```python
from build123d import *

# Parameters (mm, degrees)
SKETCH1_R           = 2.6
BOSS_EXTRUDE1_DEPTH = 5


with BuildPart() as part:
    # Sketch1 → Boss-Extrude1 (new body)
    with BuildSketch(Plane.XY):
        with BuildLine():
            Line((-144.395039413, -128.65), (-89.395039413, -128.65))
            Line((-89.395039413, -128.65), (-89.395039413, -113.602732617))
            add(Edge.make_bspline(
                [(-89.395039413, -113.602732617), (-96.831752604, -104.34489473), (-107.166514085, -96.997462442), (-119.395039413, -95.65)],
                knots=[0, 0, 0, 0, 1, 1, 1, 1], degree=3))
            Line((-119.395039413, -95.65), (-129.395039413, -95.65))
            Line((-129.395039413, -95.65), (-129.395039413, -90.65))
            Line((-129.395039413, -90.65), (-149.395039413, -90.65))
            Line((-149.395039413, -90.65), (-149.395039413, -95.65))
            Line((-149.395039413, -95.65), (-159.395039413, -95.65))
            Line((-159.395039413, -95.65), (-159.395039413, -90.65))
            Line((-159.395039413, -90.65), (-179.395039413, -90.65))
            Line((-179.395039413, -90.65), (-179.395039413, -95.65))
            add(Edge.make_bspline(
                [(-179.395039413, -95.65), (-181.601038643, -112.074647686), (-182.084492752, -128.65)],
                knots=[0, 0, 0, 1, 1, 1], degree=2))
            add(Edge.make_bspline(
                [(-182.084492752, -128.65), (-182.242729915, -142.32211305), (-189.395039413, -154.585895155)],
                knots=[0, 0, 0, 1, 1, 1], degree=2))
            Line((-189.395039413, -154.585895155), (-189.395039413, -164.35))
            Line((-189.395039413, -164.35), (-179.395039413, -164.35))
            Line((-179.395039413, -164.35), (-179.395039413, -169.35))
            Line((-179.395039413, -169.35), (-159.395039413, -169.35))
            Line((-159.395039413, -169.35), (-159.395039413, -164.35))
            Line((-159.395039413, -164.35), (-149.395039413, -164.35))
            Line((-149.395039413, -164.35), (-149.395039413, -169.35))
            Line((-149.395039413, -169.35), (-129.395039413, -169.35))
            Line((-129.395039413, -169.35), (-129.395039413, -164.35))
            Line((-129.395039413, -164.35), (-119.395039413, -164.35))
            add(Edge.make_bspline(
                [(-89.395039413, -146.397267383), (-96.831752604, -155.65510527), (-107.166514085, -163.002537558), (-119.395039413, -164.35)],
                knots=[0, 0, 0, 0, 1, 1, 1, 1], degree=3))
            Line((-89.395039413, -146.397267383), (-89.395039413, -131.35))
            Line((-89.395039413, -131.35), (-144.395039413, -131.35))
            Line((-144.395039413, -131.35), (-144.395039413, -128.65))
        make_face()
        with Locations((-104.860428981, -112.5)):
            Circle(SKETCH1_R, mode=Mode.SUBTRACT)
        with Locations((-104.860428981, -147.5)):
            Circle(SKETCH1_R, mode=Mode.SUBTRACT)
    extrude(amount=BOSS_EXTRUDE1_DEPTH)


solid = part.part
```
Read the model definition and answer for the solid it produces. Units are mm, in the model's axes. A direction names the side the tool comes from. Round coordinates to 2 decimals unless told otherwise and drop trailing zeros. One line per item, written item: value.
Q1. Which of the six approach directions +Z, -Z, +X, -X, +Y, -Y give full straight-line access (tool end or side, diameter ignored) to faces 4 (the flat face through (-124, -95.65, 2)), 5 (the flat face through (-117, -131.35, 2)), 6 (the flat face through (-179.395, -93, 2)), 7 (the flat face through (-149.395, -93, 2))?
The answers:
face 4: +Z, -Z, +X, +Y
face 5: +Z, -Z, +X
face 6: +Z, -Z, -X, +Y
face 7: +Z, -Z, +Y
Q2. Each of these flat-tipped pins is pushed along its axis until it touches: P1, Ø1, axis at y = -123.5, z = 2.5, coming from the -X side; P2, Ø1.5, axis at x = -125, z = 2, coming from the +Y side; P3, Ø4, axis at x = -104.86, y = -147.5, coming from the +Z side; P4, Ø2, axis at y = -127.5, z = 1.5, coming from the -X side. Where does it stop, or does it pass through?
The answers:
P1: stops at x = -181.91
P2: stops at y = -95.65
P3: passes through
P4: stops at x = -182.08
Q3. Find section A-A (z = 3.15). Count the separate pieces of the cut face and the enclosed holes in it, and give its area (3 significant figures).
The answers:
separate pieces: 1
enclosed holes: 2
area: 6,300 mm2
Q4. Straight lines are drawn through the part: line 1 (Y direction, x = -141, z = 3.55); line 2 (X direction, y = -166, z = 2.75); line 3 (Y direction, x = -117, z = 3.45). For each, find the intervals that lie inside material, in ascending order. Write a range as from..to.
The answers:
line 1: y = -169.35..-131.35, -128.65..-90.65
line 2: x = -179.4..-159.4, -149.4..-129.4
line 3: y = -164.01..-131.35, -128.65..-95.99
Q5. For a pull along X with two mould halves and no side action, classify faces 1 (the flat face through (-89.395, -121, 2)), 2 (the flat face through (-154, -164.35, 2)), 3 (the flat face through (-117, -128.65, 2)) as pulls with the +X half, pulls with the -X half, needs draft (parallel to the pull), parting line crosses it, or undercut.
The answers:
face 1: pulls with the +X half
face 2: undercut
face 3: needs draft
